Model file for the job. Use its own axes, mm. Round coordinates to 2 decimals unless told otherwise and drop trailing zeros. Write each loop counter-clockwise with the first axis right and the second up, starting at its lowest first coordinate (ties: lowest second). Pieces come first, ordered by that corner, then holes. Notation, with made-up numbers: (87.25, 82) - (133.25, 82) arc R12 cw to (133.25, 86) - close; hole circle Ø7 at (54.5, 1.25). An arc over 180 degrees is marked (long way). Answer as a JSON object with one key per item and string values. Group by question number.
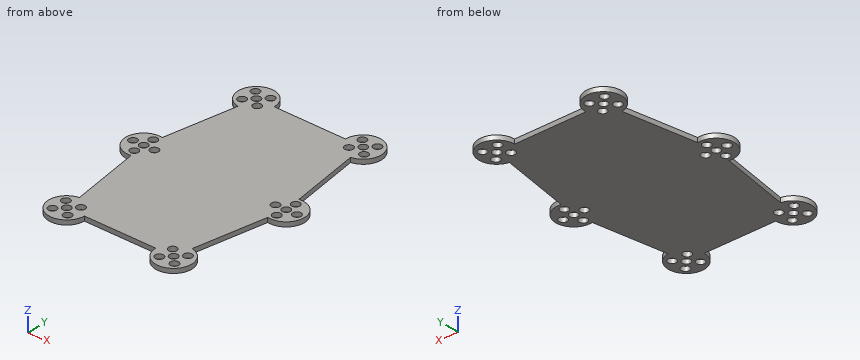
from build123d import *

# Parameters (mm, degrees)
F0_R     = 2.3
F1_DEPTH = 2.5


with BuildPart() as f1:
    # F0 (on Top) → F1 (new body)
    with BuildSketch(Plane.XY):
        with BuildLine():
            Line((-31.64399, 50.136061), (-38.35601, 9.863939))
            ThreePointArc((-38.35601, 9.863939), (-50, 0), (-38.35601, -9.863939))
            Line((-38.35601, -9.863939), (-31.64399, -50.136061))
            ThreePointArc((-31.64399, -50.136061), (-36.516243, -67.585419), (-20.000952, -60.137994))
            Line((-20.000952, -60.137994), (20.000038, -60.027598))
            ThreePointArc((20.000038, -60.027598), (36.474272, -67.621273), (31.64399, -50.136061))
            Line((31.64399, -50.136061), (38.35601, -9.863939))
            ThreePointArc((38.35601, -9.863939), (50, 0), (38.35601, 9.863939))
            Line((38.35601, 9.863939), (31.64399, 50.136061))
            ThreePointArc((31.64399, 50.136061), (36.463749, 67.6302), (20, 60))
            Line((20, 60), (-20, 60))
            ThreePointArc((-20, 60), (-36.463749, 67.6302), (-31.64399, 50.136061))
        make_face()
        with Locations((-34.242641, -64.242641)):
            Circle(F0_R, mode=Mode.SUBTRACT)
        with Locations((-25.757359, -64.242641)):
            Circle(F0_R, mode=Mode.SUBTRACT)
        with Locations((-34.242641, -55.757359)):
            Circle(F0_R, mode=Mode.SUBTRACT)
        with Locations((-30, -60)):
            Circle(F0_R, mode=Mode.SUBTRACT)
        with Locations((-25.757359, -55.757359)):
            Circle(F0_R, mode=Mode.SUBTRACT)
        with Locations((-40, -6)):
            Circle(F0_R, mode=Mode.SUBTRACT)
        with Locations((25.757359, -64.242641)):
            Circle(F0_R, mode=Mode.SUBTRACT)
        with Locations((34.242641, -64.242641)):
            Circle(F0_R, mode=Mode.SUBTRACT)
        with Locations((30, -60)):
            Circle(F0_R, mode=Mode.SUBTRACT)
        with Locations((25.757359, -55.757359)):
            Circle(F0_R, mode=Mode.SUBTRACT)
        with Locations((34.242641, -55.757359)):
            Circle(F0_R, mode=Mode.SUBTRACT)
        with Locations((40, -6)):
            Circle(F0_R, mode=Mode.SUBTRACT)
        with Locations((-46, 0)):
            Circle(F0_R, mode=Mode.SUBTRACT)
        with Locations((-40, 0)):
            Circle(F0_R, mode=Mode.SUBTRACT)
        with Locations((-40, 6)):
            Circle(F0_R, mode=Mode.SUBTRACT)
        with Locations((-34, 0)):
            Circle(F0_R, mode=Mode.SUBTRACT)
        with Locations((-34.242641, 55.757359)):
            Circle(F0_R, mode=Mode.SUBTRACT)
        with Locations((-25.757359, 55.757359)):
            Circle(F0_R, mode=Mode.SUBTRACT)
        with Locations((-30, 60)):
            Circle(F0_R, mode=Mode.SUBTRACT)
        with Locations((-34.242641, 64.242641)):
            Circle(F0_R, mode=Mode.SUBTRACT)
        with Locations((-25.757359, 64.242641)):
            Circle(F0_R, mode=Mode.SUBTRACT)
        with Locations((34, 0)):
            Circle(F0_R, mode=Mode.SUBTRACT)
        with Locations((40, 0)):
            Circle(F0_R, mode=Mode.SUBTRACT)
        with Locations((40, 6)):
            Circle(F0_R, mode=Mode.SUBTRACT)
        with Locations((46, 0)):
            Circle(F0_R, mode=Mode.SUBTRACT)
        with Locations((25.757359, 55.757359)):
            Circle(F0_R, mode=Mode.SUBTRACT)
        with Locations((30, 60)):
            Circle(F0_R, mode=Mode.SUBTRACT)
        with Locations((34.242641, 55.757359)):
            Circle(F0_R, mode=Mode.SUBTRACT)
        with Locations((25.757359, 64.242641)):
            Circle(F0_R, mode=Mode.SUBTRACT)
        with Locations((34.242641, 64.242641)):
            Circle(F0_R, mode=Mode.SUBTRACT)
    extrude(amount=F1_DEPTH)


solid = f1.part
(1) Slice it at D-D (y = -25.5). Write the cut outline in (x, z).
(2) Drill centre lines: line 1 (X direction, y = 61, z = 1.8); line 2 (Y direction, x = -24.5, z = 0.9); line 3 (Y direction, x = -39, z = 1.9). Where is each one in solid material? Low to high. Write a range as from..to.
(3) Slice it at C-C (x = 30). Write the cut outline in (y, z).
(4) Slice it at A-A (y = 6). Write the cut outline in (x, z).
(5) Slice it at B-B (x = 46). Write the cut outline in (y, z).
(6) Flat gauge pins, fed straight in: pin 1 (5.5 mm diameter, centred on x = 30, y = -60, fed in from +Z); pin 2 (1.5 mm diameter, centred on y = 48, z = 0.5, fed in from +X) (3 decimals). Where does each tip first touch, or does it go through?
Answer:
{
 "1": {"outline": "(-35.75, 0) - (35.75, 0) - (35.75, 2.5) - (-35.75, 2.5) - close"},
 "2": {"line 1": "-39.95..-32.07, -27.93..-20.05, 20.05..27.93, 32.07..39.95", "line 2": "-68.35..-66.17, -62.32..-57.68, -53.83..53.83, 57.68..62.32, 66.17..68.35", "line 3": "-64.36..-55.64, -9.95..-8.07, -3.93..-2.07, 2.07..3.93, 8.07..9.95, 55.64..64.36"},
 "3": {"outline": "(-70, 0) - (-62.3, 0) - (-62.3, 2.5) - (-70, 2.5) - close; (-57.7, 0) - (57.7, 0) - (57.7, 2.5) - (-57.7, 2.5) - close; (62.3, 0) - (70, 0) - (70, 2.5) - (62.3, 2.5) - close"},
 "4": {"outline": "(-48, 0) - (-42.3, 0) - (-42.3, 2.5) - (-48, 2.5) - close; (-37.7, 0) - (37.7, 0) - (37.7, 2.5) - (-37.7, 2.5) - close; (42.3, 0) - (48, 0) - (48, 2.5) - (42.3, 2.5) - close"},
 "5": {"outline": "(-8, 0) - (-2.3, 0) - (-2.3, 2.5) - (-8, 2.5) - close; (2.3, 0) - (8, 0) - (8, 2.5) - (2.3, 2.5) - close"},
 "6": {"pin 1": "z = 2.5", "pin 2": "x = 32.125"}
}
